The listing builds one solid part. Answer for the finished solid, in the listing's coordinates (mm). Face numbers are marked on the shaded views. Round coordinates to 2 decimals unless told otherwise and drop trailing zeros. Write each loop counter-clockwise with the first axis right and the second up, starting at its lowest first coordinate (ties: lowest second). Pieces come first, ordered by that corner, then holes.
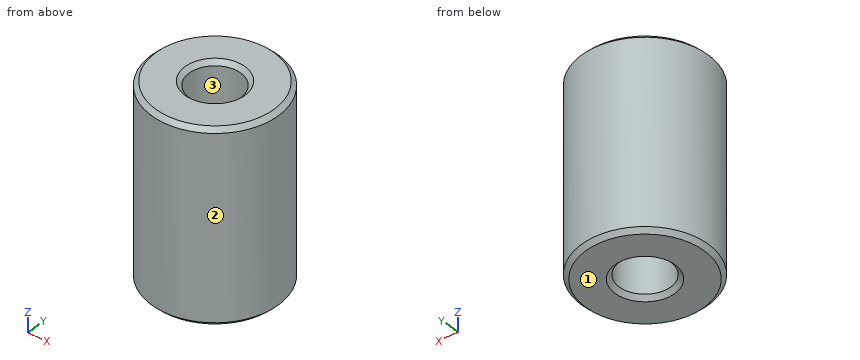
from build123d import *

# Parameters (mm, degrees)
SZKIC1_R                    = 15
SZKIC1_R_2                  = 6.1
DODANIE_WYCI_GNI_CIE1_DEPTH = 45
SFAZOWANIE1_SIZE            = 1


with BuildPart() as part:
    # Szkic1 → Dodanie-wyciągnięcie1 (new body)
    with BuildSketch(Plane.XY):
        Circle(SZKIC1_R)
        Circle(SZKIC1_R_2, mode=Mode.SUBTRACT)
    extrude(amount=DODANIE_WYCI_GNI_CIE1_DEPTH)

    # Sfazowanie1
    sfazowanie1_edges = [part.edges().sort_by_distance(p)[0] for p in [
        (-15, 0, 0),
        (-15, 0, 45),
        (-6.1, 0, 0),
        (-6.1, 0, 45),
    ]]
    chamfer(sfazowanie1_edges, length=SFAZOWANIE1_SIZE)


solid = part.part
1. Section C-C on z = 41 is taken. Determine the outline of the cut face in (x, y).
Geometry says:
outline: circle Ø30 at (0, 0); hole circle Ø12.2 at (0, 0)
2. Straight lines are drawn through the part: line 1 along Y through (x, z) = (0, 31); line 2 along X through (y, z) = (3, 23); line 3 along Y through (x, z) = (5, 39). For each, find the intervals that lie inside material, in ascending order.
Geometry says:
line 1: y = -15 to -6.1, 6.1 to 15
line 2: x = -14.7 to -5.31, 5.31 to 14.7
line 3: y = -14.14 to -3.49, 3.49 to 14.14
3. Section A-A on y = 0 is taken. Determine the outline of the cut face in (x, z), plus the area to 3 significant figures.
Geometry says:
outline: (-15, 1) - (-14, 0) - (-7.1, 0) - (-6.1, 1) - (-6.1, 44) - (-7.1, 45) - (-14, 45) - (-15, 44) - close; (6.1, 1) - (7.1, 0) - (14, 0) - (15, 1) - (15, 44) - (14, 45) - (7.1, 45) - (6.1, 44) - close
area: 797 mm2
4. For a pull along Y with two mould halves and no side action, classify the marked faces 1, 2 and 3 as released by +Y, released by -Y, zero draft, split by the parting line, or undercut.
Geometry says:
face 1: zero draft
face 2: split by the parting line
face 3: undercut
5. Given pin 1 (14 mm diameter, centred on x = 0, y = 0, fed in from -Z); pin 2 (4 mm diameter, centred on x = -8.5, z = 18.5, fed in from -Y); pin 3 (10 mm diameter, centred on x = -7.5, z = 23, fed in from -Y), each flat-ended and moving along its own axis, determine where each tip first touches the part or whether it passes through.
Geometry says:
pin 1: stops at z = 0.1
pin 2: stops at y = -13.52
pin 3: stops at y = -14.79
